```python
from build123d import *

# Parameters (mm, degrees)
BOSS_EXTRUDE1_DEPTH        = 2.54
FILLET3_R                  = 25.4
F_10_CLEARANCE_HOLE1_D     = 5.1054
F_10_CLEARANCE_HOLE1_DEPTH = 9.906
F_10_CLEARANCE_HOLE1_TIP   = 1.533816902
FILLET4_R                  = 25.4


with BuildPart() as part:
    # Sketch1 → Boss-Extrude1 (new body)
    with BuildSketch(Plane(origin=(0, 0, 0), x_dir=(1, 0, 0), z_dir=(0, 1, 0))):
        Polygon((38.706788555, 38.706788555), (79.551048595, 79.551048595), (100.554615109, 152.799189826), (89.598560117, 196.741526293), (64.953048669, 190.596710145), (74.170272892, 153.628442974), (56.667300797, 92.588325282), (20.746276313, 56.667300797), (-46.605644595, 25.236404374), (7.275892132, -28.645132353), align=None)
        Polygon((8.285025385, 20.746276313), (5.535394728, 25.508776313), (0.036133414, 25.508776313), (-2.713497243, 20.746276313), (0.036133414, 15.983776313), (5.535394728, 15.983776313), align=None, mode=Mode.SUBTRACT)
    extrude(amount=BOSS_EXTRUDE1_DEPTH)

    # Fillet3
    fillet3_edges = [part.edges().sort_by_distance(p)[0] for p in [
        (64.953048669, 1.27, -190.596710145),
    ]]
    fillet(fillet3_edges, radius=FILLET3_R - 0.0001)  # a hair under: the kernel refuses the full size

    # #10 Clearance Hole1
    with Locations(Plane(origin=(0, 2.54, 0), x_dir=(1, 0, 0), z_dir=(0, 1, 0))):
        with Locations((84.531663752, 177.691526293), (87.362444, 153.2138164), (77.735809348, 119.641751669), (68.109174696, 86.069686939), (48.917853565, 66.878365807)):
            Hole(F_10_CLEARANCE_HOLE1_D / 2, depth=F_10_CLEARANCE_HOLE1_DEPTH)
            with Locations((0, 0, -(F_10_CLEARANCE_HOLE1_DEPTH + F_10_CLEARANCE_HOLE1_TIP / 2))):  # 118° drill point
                Cone(0, F_10_CLEARANCE_HOLE1_D / 2, F_10_CLEARANCE_HOLE1_TIP, mode=Mode.SUBTRACT)

    # Fillet4
    fillet4_edges = [part.edges().sort_by_distance(p)[0] for p in [
        (7.275892132, 1.27, 28.645132353),
        (-46.605644595, 1.27, -25.236404374),
    ]]
    fillet(fillet4_edges, radius=FILLET4_R)


solid = part.part
```
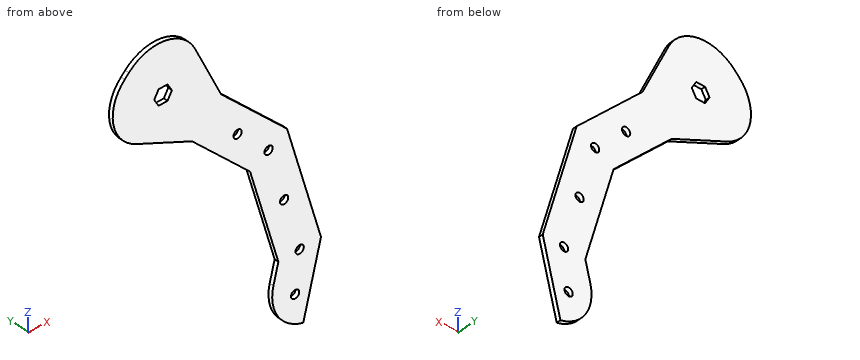
Verification items for the finished model (mm, model axes). Coordinates: 2 decimals unless noted, no trailing zeros. Loops run counter-clockwise (first coordinate to the right, second up) from the corner with the lowest first, then second, coordinate; pieces in that order, holes last. Notation, with made-up numbers: (33, -2.75) - (67, -2.75) arc R9 cw to (67, 1.25) - close; hole circle Ø9 at (56.5, -29). An arc over 180 degrees is marked (long way). Answer as a JSON object with one key per item and string values.
(1) Scan lines: line 1 along X through (y, z) = (0.2, -152); line 2 along X through (y, z) = (1.45, -68); line 3 along X through (y, z) = (1.2, -113). Record each from-to range of solid material in increasing order.
Response:
{"line 1": "x = 73.7 to 85.12, 89.61 to 100.33", "line 2": "x = 32.08 to 46.62, 51.21 to 68", "line 3": "x = 62.52 to 89.14"}
(2) Cross-section at C-C, the plane z = -160. Record the boundary of the cut face in (x, y).
Response:
{"outline": "(72.58, 0) - (98.76, 0) - (98.76, 2.54) - (72.58, 2.54) - close"}
(3) Cross-section at B-B, the plane z = -72.5. Record the boundary of the cut face in (x, y).
Response:
{"outline": "(36.58, 0) - (72.5, 0) - (72.5, 2.54) - (36.58, 2.54) - close"}
(4) Go/stop test with a flat-tipped pin: pin 1 Ø1.5 at (x, y) = (1.5, 1) entering from +Z. Record where the tip stops, or that it passes through.
Response:
{"pin 1": "stops at z = 10.42"}
(5) Cross-section at A-A, the plane y = 1.7. Count the separate pieces of the cut face and the enclosed holes in it, then the cut area to 3 significant figures.
Response:
{"separate pieces": "1", "enclosed holes": "6", "area": "6,850 mm²"}
